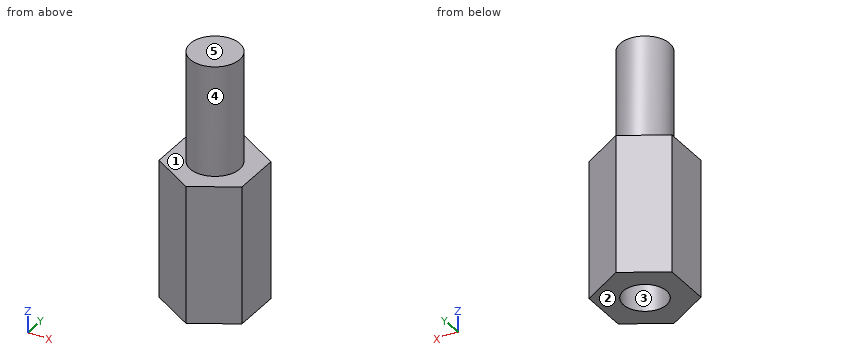
Autodesk Inventor part; units mm, degrees
ref_plane "YZ Plane" through (0, 0, 0) normal (1, 0, 0) x (0, 1, 0)
ref_plane "XZ Plane" through (0, 0, 0) normal (0, 1, 0) x (-1, 0, 0)
ref_plane "XY Plane" through (0, 0, 0) normal (0, 0, 1) x (1, 0, 0)
sketch "Sketch1" plane through (0, 0, 0) normal (0, 0, 1) x (1, 0, 0)
  line L0 (1.5, 0.866) -> (1.5, -0.866)
  line L1 (1.5, -0.866) -> (0, -1.732)
  line L2 (0, -1.732) -> (-1.5, -0.866)
  line L3 (-1.5, 0.866) -> (-1.5, -0.866)
  line L4 (-1.5, 0.866) -> (0, 1.732)
  line L5 (0, 1.732) -> (1.5, 0.866)
  circle A0 centre (0, 0) radius 1.732 construction
  line L6 (0, 30.018) -> (0, -6.2677) construction
  line L7 (0, -13.5249) -> (0, 37.2751)
  line L8 (-2.4248, 0) -> (2.4248, 0)
  dimension "d0" = 3.464
  dimension "d20" = 2.9999
  dimension "d21" = 1.732
extrude "Hexagon1" add sketch "Sketch1" along normal blind 5
hole "Hole1" at (0, 0, 0) direction (0, 0, 1) diameter 1.567 depth 4
sketch "Sketch2" plane through (0, 0, 5) normal (0, 0, 1) x (1, 0, 0)
  circle A0 centre (0, 0) radius 0.9
  dimension "d22" = 1.8
extrude "Extrusion2" add sketch "Sketch2" along normal blind 4
thread "Thread3"
properties part number "Spacer-M2-05" material "Brass, Soft Yellow, Welded"
The listing builds one solid part. Answer for the finished solid, in the listing's coordinates (mm). Face numbers are marked on the shaded views. A direction names the side the tool comes from. Give positions to 0.01 mm unless a question says otherwise; leave off trailing zeros. Write each loop counter-clockwise with the first axis right and the second up, starting at its lowest first coordinate (ties: lowest second). Pieces come first, ordered by that corner, then holes.
1) A tool of negligible diameter and unlimited length cuts with its end or side. For the marked faces 1 and 2, from which of +Z, -Z, +X, -X, +Y, -Y can it reach the whole face along a straight path? Write none if from no direction.
2) Section B-B (y = 0) is taken. Write down the section's boundary in (x, z), and give its area (3 significant figures).
3) Section D-D (z = 8) is taken. Write down the section's boundary in (x, y).
4) For a pull along Y with two mould halves and no side action, classify the marked faces 3, 4 and 5 as pulls with the +Y half, pulls with the -Y half, needs draft (parallel to the pull), parting line crosses it, or undercut.
5) Section C-C (x = -0.3) is taken. Write down the section's boundary in (y, z), and give its area (3 significant figures).
6) Given P1, Ø1, axis at y = 0.5, z = 7.5, coming from the +X side; P2, Ø1, axis at x = -1, z = 1.5, coming from the +Y side, each flat-ended and moving along its own axis, determine where each tip first touches the part or whether it passes through.
7) Find the intervals of material crossed by L1, parallel to X at y = 0, z = 3.05; L2, parallel to Z at x = 0.85, y = -1; L3, parallel to Z at x = 0.2, y = -0.4, in increasing order.
8) Section A-A (z = 3.5) is taken. Write down the section's boundary in (x, y).
Response:
1. face 1: +Z
1. face 2: -Z, +X, -X, +Y, -Y
2. outline: (-1.5, 0) - (-0.78, 0) - (-0.78, 4) - (0.78, 4) - (0.78, 0) - (1.5, 0) - (1.5, 5) - (0.9, 5) - (0.9, 9) - (-0.9, 9) - (-0.9, 5) - (-1.5, 5) - close
2. area: 15.9 mm2
3. outline: circle Ø1.8 at (0, 0)
4. face 3: undercut
4. face 4: parting line crosses it
4. face 5: needs draft
5. outline: (-1.56, 0) - (-0.72, 0) - (-0.72, 4) - (0.72, 4) - (0.72, 0) - (1.56, 0) - (1.56, 5) - (0.85, 5) - (0.85, 9) - (-0.85, 9) - (-0.85, 5) - (-1.56, 5) - close
5. area: 16.6 mm2
6. P1: stops at x = 0.9
6. P2: stops at y = 1.44
7. L1: x = -1.5 to -0.78, 0.78 to 1.5
7. L2: z = 0 to 5
7. L3: z = 4 to 9
8. outline: (-1.5, -0.87) - (0, -1.73) - (1.5, -0.87) - (1.5, 0.87) - (0, 1.73) - (-1.5, 0.87) - close; hole circle Ø1.57 at (0, 0)
